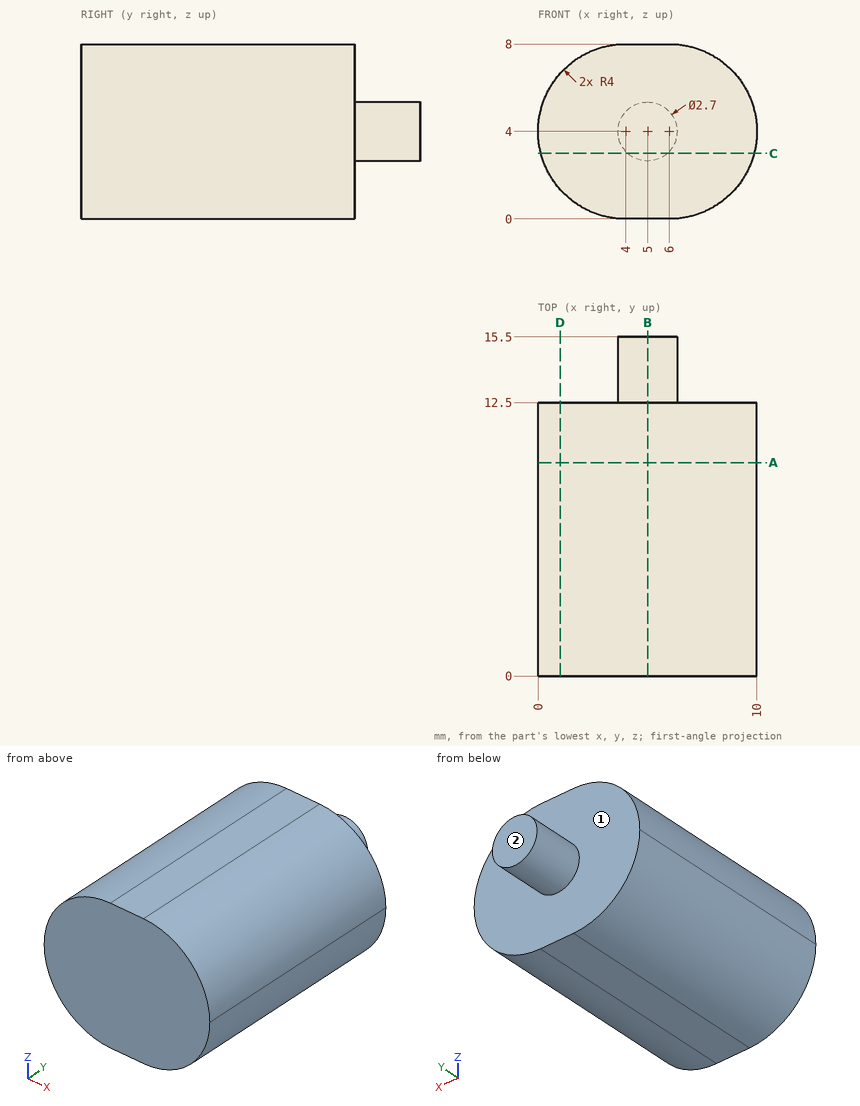
Study the drawing (mm; zero at the part's minimum x, y, z) and answer. A direction names the side the tool comes from. Round coordinates to 2 decimals unless told otherwise and drop trailing zeros. Write each loop counter-clockwise with the first axis right and the second up, starting at its lowest first coordinate (ties: lowest second). Pieces come first, ordered by that corner, then holes. Notation, with made-up numbers: (73, -1.75) -> (114, -1.75) arc R22 cw to (114, 10.25) -> close; hole circle Ø4 at (7.5, 4.25). An arc over 180 degrees is marked (long way). Write item = value, one per line.
1) Section D-D on x = 1 is taken. Write down the section's boundary in (y, z), plus the area to 3 significant figures.
Check values:
outline = (0, 1.35) -> (12.5, 1.35) -> (12.5, 6.65) -> (0, 6.65) -> close
area = 66.1 mm²
2) Section B-B on x = 5 is taken. Write down the section's boundary in (y, z), plus the area to 3 significant figures.
Check values:
outline = (0, 0) -> (12.5, 0) -> (12.5, 2.65) -> (15.5, 2.65) -> (15.5, 5.35) -> (12.5, 5.35) -> (12.5, 8) -> (0, 8) -> close
area = 108 mm²
3) Which of the six approach directions +Z, -Z, +X, -X, +Y, -Y give full straight-line access (tool end or side, diameter ignored) to the marked faces 1 and 2?
Check values:
face_1 = +Y
face_2 = +Z, -Z, +X, -X, +Y
4) Section A-A on y = 9.75 is taken. Write down the section's boundary in (x, z).
Check values:
outline = (4, 0) -> (6, 0) arc R4 ccw to (6, 8) -> (4, 8) arc R4 ccw to start
5) Straight lines are drawn through the part: line 1 along Y through (x, z) = (1.75, 1.75); line 2 along Z through (x, y) = (3, 5.75); line 3 along Z through (x, y) = (8.5, 6.5). For each, find the intervals that lie inside material, in ascending order. Write a range as [from, to].
Check values:
line_1 = [0, 12.5]
line_2 = [0.13, 7.87]
line_3 = [0.88, 7.12]
6) Given pin 1 (3 mm diameter, centred on x = 2.5, z = 1.5, fed in from +Y); pin 2 (1 mm diameter, centred on x = 3, y = 11, fed in from +Z); pin 3 (2 mm diameter, centred on x = 8, y = 10.5, fed in from +Z), each flat-ended and moving along its own axis, determine where each tip first touches the part or whether it passes through.
Check values:
pin_1 = 12.5
pin_2 = 7.97
pin_3 = 7.87
7) Section C-C on z = 3 is taken. Write down the section's boundary in (x, y).
Check values:
outline = (0.13, 0) -> (9.87, 0) -> (9.87, 12.5) -> (5.91, 12.5) -> (5.91, 15.5) -> (4.09, 15.5) -> (4.09, 12.5) -> (0.13, 12.5) -> close
